Autodesk Fusion 360 part; units mm, degrees
sketch "Esquisse1" plane through (0, 0, 0) normal (0, 0, 1) x (1, 0, 0)
  line L0 (0, 0) -> (60, 0)
  line L1 (60, 0) -> (60, 45)
  line L2 (60, 45) -> (0, 45)
  line L3 (0, 45) -> (0, 0)
  dimension "d1" = 60
  dimension "d2" = 45
extrude "Extrusion1" add sketch "Esquisse1" along normal blind 2.5
fillet "Congé1" radius 7 1 edges at (60, 0, 1.25)
sketch "Esquisse2" plane through (0, 0, 2.5) normal (0, 0, 1) x (-1, 0, 0)
  arc A0 (-53, 0) -> (-60, -7) centre (-53, -7) ccw
  line L0 (-60, -7) -> (-60, -45)
  line L1 (-60, -45) -> (0, -45)
  line L2 (0, -45) -> (0, 0)
  line L3 (0, 0) -> (-53, 0)
  line L4 (-36.0159, -29.1423) -> (-49.0159, -29.1423)
  line L5 (-49.0159, -29.1423) -> (-49.0159, -16.1423)
  line L6 (-49.0159, -16.1423) -> (-36.0159, -16.1423)
  line L7 (-36.0159, -16.1423) -> (-36.0159, -29.1423)
  dimension "d7" = 13
  dimension "d8" = 13
extrude "Extrusion2" cut sketch "Esquisse2" against normal blind 2.5 contours L4 L5 L6 L7
sketch "Esquisse3" plane through (0, 0, 2.5) normal (0, 0, 1) x (-1, 0, 0)
  line L0 (-49.0159, -29.1423) -> (-49.0159, -16.1423)
  line L1 (-49.0159, -16.1423) -> (-36.0159, -16.1423)
  line L2 (-36.0159, -16.1423) -> (-36.0159, -29.1423)
  line L3 (-36.0159, -29.1423) -> (-49.0159, -29.1423)
  arc A0 (-53, 0) -> (-60, -7) centre (-53, -7) ccw
  line L4 (-60, -7) -> (-60, -45)
  line L5 (-60, -45) -> (0, -45)
  line L6 (0, -45) -> (0, 0)
  line L7 (0, 0) -> (-53, 0)
  circle A1 centre (-19, -23) radius 10.5
  dimension "d11" = 21
extrude "Extrusion3" cut sketch "Esquisse3" against normal blind 2.5 contours A1
Source: CAD feature listing. Evaluate the final solid. Frame: model axes, mm. A direction names the side the tool comes from. Round coordinates to 2 decimals unless told otherwise and drop trailing zeros. Order: outer loops, then holes, each group sorted by start corner. A loop starts at its lowest first (then second) coordinate and runs counter-clockwise, first axis right, second up. Notation, with made-up numbers: (59, -15.75) - (112, -15.75) arc R35 ccw to (112, 20.25) - close; hole circle Ø3 at (-38.5, 32.5). An arc over 180 degrees is marked (long way). Use a Markdown table: item, result. Add a question column.
1. Section query D-D (x = 42). Return the cut outline in (y, z), then the cut area to 3 significant figures.
2. Section query C-C (z = 0.4). Return the cut outline in (x, y).
3. Section query A-A (x = 19). Return the cut outline in (y, z), then the cut area to 3 significant figures.
4. Set-up query: faces 1 (the cylindrical face through (57.9, 2, 1.3)), 2 (the flat face through (42, 29.142, 1)). Return all of +Z, -Z, +X, -X, +Y, -Y with unobstructed straight access to the full face (end or side cutting, diameter ignored); none if empty.
5. Section query B-B (y = 23). Return the cut outline in (x, z).
6. Mould query, pull axis X, two halves, no side actions, for faces 3 (the flat face through (30, 23, 2.5)), 4 (the flat face through (36.016, 23, 1)), 5 (the flat face through (43, 16.142, 1)), 6 (the flat face through (60, 26, 1)). Classes: +X half, -X half, draft (parallel to the pull), parting line (faces both ways), or undercut.
7. Line query: probe 1 along X at (y, z) = (23, 1.7); probe 2 along Y at (x, z) = (19, 0.95); probe 3 along X at (y, z) = (21, 1.4). Output: solid intervals per line, ascending.
Derived:
| question | item | result |
|---|---|---|
| 1 | outline | (0, 0) - (16.14, 0) - (16.14, 2.5) - (0, 2.5) - close; (29.14, 0) - (45, 0) - (45, 2.5) - (29.14, 2.5) - close |
| 1 | area | 80.0 mm2 |
| 2 | outline | (0, 0) - (53, 0) arc R7 ccw to (60, 7) - (60, 45) - (0, 45) - close; hole circle Ø21 at (19, 23); hole (36.02, 16.14) - (49.02, 16.14) - (49.02, 29.14) - (36.02, 29.14) - close |
| 3 | outline | (0, 0) - (12.5, 0) - (12.5, 2.5) - (0, 2.5) - close; (33.5, 0) - (45, 0) - (45, 2.5) - (33.5, 2.5) - close |
| 3 | area | 60.0 mm2 |
| 4 | face 1 | +Z, -Z, +X, -Y |
| 4 | face 2 | +Z, -Z |
| 5 | outline | (0, 0) - (8.5, 0) - (8.5, 2.5) - (0, 2.5) - close; (29.5, 0) - (36.02, 0) - (36.02, 2.5) - (29.5, 2.5) - close; (49.02, 0) - (60, 0) - (60, 2.5) - (49.02, 2.5) - close |
| 6 | face 3 | draft |
| 6 | face 4 | undercut |
| 6 | face 5 | undercut |
| 6 | face 6 | +X half |
| 7 | probe 1 | 0 to 8.5, 29.5 to 36.02, 49.02 to 60 |
| 7 | probe 2 | 0 to 12.5, 33.5 to 45 |
| 7 | probe 3 | 0 to 8.69, 29.31 to 36.02, 49.02 to 60 |
